Could you check a few things on this model? Use its own coordinates, in mm. A direction names the side the tool comes from. Give positions to 0.01 mm unless a question says otherwise; leave off trailing zeros. Loops run counter-clockwise (first coordinate to the right, second up) from the corner with the lowest first, then second, coordinate; pieces in that order, holes last.
1. Imagine slicing it at A-A (z = 12). List the corners of the cut face in (x, y) for me.
2. For faces 5 (the cylindrical face through (-20.35, 0.07, -2.54)), 6 (the cylindrical face through (-31.232, 4.101, -40.552)), which set-ups out of +Z, -Z, +X, -X, +Y, -Y let a thin tool reach every point of the face, with its end or its side?
3. Thinking about a two-plate mould opening in X: for faces 1 (the cylindrical face through (23.65, 0.07, -2.54)), 2 (the cylindrical face through (3.905, 0.867, 13.619)), 3 (the cylindrical face through (13.476, -0.632, -2.535)), 4 (the flat face through (-6.5, 6.5, 0)), which applies, +X half, -X half, draft (parallel to the pull), parting line (faces both ways), or undercut?
4. Imagine slicing it at B-B (z = -49.5). List the corners of the cut face in (x, y) for me.
5. For P1, Ø6, axis at x = 22, z = -58.5, coming from the +Y side; P2, Ø4.5, axis at x = 0, y = -22, coming from the -Z side; P3, Ø5.5, axis at x = -15, y = 0, coming from the +Z side, each with a flat end and sliding along its axis, tell me the tip position at first contact or that it passes through.
6. I need wall thicknesses on line 1 along X through (y, z) = (0, -3); line 2 along Z through (x, y) = (-15.5, -13); line 3 along Z through (x, y) = (-7.5, -3). Which ranges of each line are inside material? Lowest first, please.
```python
from build123d import *

# Parameters (mm, degrees)
TAP_DRILL_FOR_M4X0_7_TAP1_D     = 3.3
TAP_DRILL_FOR_M4X0_7_TAP1_DEPTH = 5
TAP_DRILL_FOR_M4X0_7_TAP1_TIP   = 0.991420021


with BuildPart() as part:
    # Sketch2 → Revolve1 (revolve)
    with BuildSketch(Plane(origin=(0, 0, 0), x_dir=(0, 0, -1), z_dir=(1, 0, 0)), mode=Mode.PRIVATE) as revolve1_sk:
        Polygon((2, 0), (2, 5), (-5, 5), (-5, 4), (-22, 4), (-22, 3.8), (-23, 3.8), (-23, 4), (-24, 4), (-24, 0), align=None)
        Polygon((2, 9), (2, 0), (74, 0), (74, 15), (73, 15), (73, 31.5), (9, 31.5), (0, 27.5), (0, 9), align=None)
    revolve(revolve1_sk.sketch.rotate(Axis((0, 0, -2), (0, 0, -1)), 180), axis=Axis((0, 0, -2), (0, 0, -1)))

    # Tap Drill for M4x0.7 Tap1
    with Locations(Plane(origin=(0, 22, 0), x_dir=(1, 0, 0), z_dir=(0, 0, 1))):
        with Locations((0, 0), (0, -7), (15, -22), (22, -22), (0, -37), (0, -44), (-15, -22), (-22, -22)):
            Hole(TAP_DRILL_FOR_M4X0_7_TAP1_D / 2, depth=TAP_DRILL_FOR_M4X0_7_TAP1_DEPTH)
            with Locations((0, 0, -(TAP_DRILL_FOR_M4X0_7_TAP1_DEPTH + TAP_DRILL_FOR_M4X0_7_TAP1_TIP / 2))):  # 118° drill point
                Cone(0, TAP_DRILL_FOR_M4X0_7_TAP1_D / 2, TAP_DRILL_FOR_M4X0_7_TAP1_TIP, mode=Mode.SUBTRACT)


solid = part.part
```
Derived:
1. outline: circle Ø8 at (0, 0)
2. face 5: +Z
2. face 6: +Z, -Z
3. face 1: undercut
3. face 2: parting line
3. face 3: undercut
3. face 4: draft
4. outline: circle Ø63 at (0, 0)
5. P1: stops at y = 25.12
5. P2: stops at z = -73
5. P3: stops at z = 0
6. line 1: x = -28.83 to -23.65, -20.35 to -16.65, -13.35 to 13.35, 16.65 to 20.35, 23.65 to 28.83
6. line 2: z = -73 to 0
6. line 3: z = -74 to -2
